CAD build for the part. Positions are in the model's coordinates, mm. A direction names the side the tool comes from. Give positions to 0.01 mm unless a question says otherwise; leave off trailing zeros. Loops run counter-clockwise (first coordinate to the right, second up) from the corner with the lowest first, then second, coordinate; pieces in that order, holes last. Notation, with made-up numbers: M 38.25,7 L 64.25,7 A27 cw 64.25,25 Z; hole C 44.5,53 d4. An arc over 180 degrees is marked long. Answer as CSV lines item,"result".
from build123d import *

# Parameters (mm, degrees)
SKETCH_W        = 43.2
SKETCH_H        = 46
SKETCH_W_2      = 31.5
SKETCH_H_2      = 34
PAD_DEPTH       = 41
SKETCH001_W     = 43.2
SKETCH001_H     = 46
SKETCH001_W_2   = 39.6
SKETCH001_H_2   = 42.4
PAD001_DEPTH    = 30
POCKET_DEPTH    = 5
SKETCH003_W     = 14
SKETCH003_H     = 12
PAD002_DEPTH    = 14
FILLET_R        = 6.99
POCKET001_DEPTH = 10
POCKET002_DEPTH = 43.201
SKETCH006_R     = 2
POCKET003_DEPTH = 2.001
SKETCH007_W     = 14
SKETCH007_H     = 12
PAD003_DEPTH    = 14
FILLET001_R     = 6.99
POCKET004_DEPTH = 10
POCKET005_DEPTH = 43.201
SKETCH010_R     = 2
POCKET006_DEPTH = 2.001


with BuildPart() as part:
    # Sketch → Pad (new body)
    with BuildSketch(Plane.XY):
        Rectangle(SKETCH_W, SKETCH_H)
        Rectangle(SKETCH_W_2, SKETCH_H_2, mode=Mode.SUBTRACT)
    extrude(amount=PAD_DEPTH)

    # Sketch001 → Pad001 (new body)
    with BuildSketch(Plane.XY.offset(41)):
        Rectangle(SKETCH001_W, SKETCH001_H)
        Rectangle(SKETCH001_W_2, SKETCH001_H_2, mode=Mode.SUBTRACT)
    extrude(amount=PAD001_DEPTH)

    # Sketch002 → Pocket (cut)
    with BuildSketch(Plane(origin=(-21.6, 0, 0), x_dir=(0, -1, 0), z_dir=(-1, 0, 0))):
        with BuildLine():
            Line((-11.5, 71), (11.5, 71))
            Line((11.5, 71), (11.5, 62.000009))
            ThreePointArc((-11.5, 61.999999), (5e-06, 50.5), (11.5, 62.000009))
            Line((-11.5, 61.999999), (-11.5, 71))
        make_face()
    extrude(amount=-POCKET_DEPTH, mode=Mode.SUBTRACT)

    # Sketch003 → Pad002 (new body)
    with BuildSketch(Plane.XZ.offset(23)):
        with Locations((-14.6, 6)):
            Rectangle(SKETCH003_W, SKETCH003_H)
        with Locations((14.6, 6)):
            Rectangle(SKETCH003_W, SKETCH003_H)
    extrude(amount=PAD002_DEPTH)

    # Fillet
    fillet_edges = [part.edges().sort_by_distance(p)[0] for p in [
        (-21.6, -37, 6),
        (-7.6, -37, 6),
        (7.6, -37, 6),
        (21.6, -37, 6),
    ]]
    fillet(fillet_edges, radius=FILLET_R)

    # Sketch004 → Pocket001 (cut)
    with BuildSketch(Plane.XY.offset(12)):
        with BuildLine():
            Line((-19.6, -23), (-9.6, -23))
            Line((-9.6, -23), (-9.6, -30.009996))
            ThreePointArc((-19.6, -30.009995), (-14.6, -35.009995), (-9.6, -30.009996))
            Line((-19.6, -30.009995), (-19.6, -23))
        make_face()
        with BuildLine():
            Line((9.6, -23), (19.6, -23))
            Line((19.6, -23), (19.6, -30.009994))
            ThreePointArc((9.6, -30.009994), (14.6, -35.009995), (19.6, -30.009994))
            Line((9.6, -30.009994), (9.6, -23))
        make_face()
    extrude(amount=-POCKET001_DEPTH, mode=Mode.SUBTRACT)

    # Sketch005 → Pocket002 (cut, through all)
    with BuildSketch(Plane(origin=(-21.6, 0, 0), x_dir=(0, -1, 0), z_dir=(-1, 0, 0))):
        Polygon((23, 12), (37, 2), (37, 12), align=None)
    extrude(amount=-POCKET002_DEPTH, mode=Mode.SUBTRACT)

    # Sketch006 → Pocket003 (cut, through all)
    with BuildSketch(Plane.XY.offset(2)):
        with Locations((-14.6, -30.009995)):
            Circle(SKETCH006_R)
        with Locations((14.6, -30.009995)):
            Circle(SKETCH006_R)
    extrude(amount=-POCKET003_DEPTH, mode=Mode.SUBTRACT)

    # Sketch007 → Pad003 (new body)
    with BuildSketch(Plane(origin=(0, 23, 0), x_dir=(-1, 0, 0), z_dir=(0, 1, 0))):
        with Locations((-14.6, 6)):
            Rectangle(SKETCH007_W, SKETCH007_H)
        with Locations((14.6, 6)):
            Rectangle(SKETCH007_W, SKETCH007_H)
    extrude(amount=PAD003_DEPTH)

    # Fillet001
    fillet001_edges = [part.edges().sort_by_distance(p)[0] for p in [
        (21.6, 37, 6),
        (7.6, 37, 6),
        (-7.6, 37, 6),
        (-21.6, 37, 6),
    ]]
    fillet(fillet001_edges, radius=FILLET001_R)

    # Sketch008 → Pocket004 (cut)
    with BuildSketch(Plane.XY.offset(12)):
        with BuildLine():
            Line((-19.6, 23), (-9.6, 23))
            Line((-9.6, 23), (-9.6, 30.009983))
            ThreePointArc((-9.6, 30.009983), (-14.6, 35.009995), (-19.6, 30.009983))
            Line((-19.6, 30.009983), (-19.6, 23))
        make_face()
        with BuildLine():
            Line((19.6, 30.009983), (19.6, 23))
            Line((19.6, 23), (9.6, 23))
            Line((9.6, 23), (9.6, 30.009983))
            ThreePointArc((19.6, 30.009983), (14.6, 35.009995), (9.6, 30.009983))
        make_face()
    extrude(amount=-POCKET004_DEPTH, mode=Mode.SUBTRACT)

    # Sketch009 → Pocket005 (cut, through all)
    with BuildSketch(Plane(origin=(-21.6, 0, 0), x_dir=(0, -1, 0), z_dir=(-1, 0, 0))):
        Polygon((-23, 12), (-37, 2), (-37, 12), align=None)
    extrude(amount=-POCKET005_DEPTH, mode=Mode.SUBTRACT)

    # Sketch010 → Pocket006 (cut, through all)
    with BuildSketch(Plane.XY.offset(2)):
        with Locations((-14.6, 30.009995)):
            Circle(SKETCH010_R)
        with Locations((14.6, 30.009995)):
            Circle(SKETCH010_R)
    extrude(amount=-POCKET006_DEPTH, mode=Mode.SUBTRACT)


solid = part.part
1) Band-saw the part on A-A on y = 0. Give the cut face in (x, z), and give its area (3 significant figures).
Answer below:
outline,"M -21.6,0 L -15.75,0 L -15.75,41 L -19.8,41 L -19.8,50.5 L -21.6,50.5 Z; M 15.75,0 L 21.6,0 L 21.6,71 L 19.8,71 L 19.8,41 L 15.75,41 Z"
area,"551 mm^2"
2) Flat gauge pins, fed straight in: pin 1 (2 mm diameter, centred on x = 4, z = 54, fed in from -Y); pin 2 (4.5 mm diameter, centred on x = -14.6, y = 30.01, fed in from +Z); pin 3 (3 mm diameter, centred on x = 14.6, y = 30.01, fed in from +Z); pin 4 (6 mm diameter, centred on x = -1.5, y = -17.5, fed in from +Z). Where does each tip first touch, or does it go through?
Answer below:
pin 1,"stops at y = -23"
pin 2,"stops at z = 2"
pin 3,"passes through"
pin 4,"stops at z = 41"
3) Mould opens along X. For faces 4 (the face through (7.6, 26, 5)), 5 (the face through (-13.525, 31.696, 1.014)), 6 (the face through (19.753, 31.004, 6.283)), 7 (the face through (20.38, 33.956, 1.991)) say: +X half, -X half, draft (parallel to the pull), parting line (faces both ways), or undercut.
Answer below:
face 4,"undercut"
face 5,"undercut"
face 6,"draft"
face 7,"+X half"
4) Band-saw the part on C-C on z = 14. Give the cut face in (x, y), and give its area (3 significant figures).
Answer below:
outline,"M -21.6,-23 L 21.6,-23 L 21.6,23 L -21.6,23 Z; hole M -15.75,-17 L 15.75,-17 L 15.75,17 L -15.75,17 Z"
area,"916 mm^2"
5) Band-saw the part on D-D on y = -19.5. Give the cut face in (x, z), and give its area (3 significant figures).
Answer below:
outline,"M -21.6,0 L 21.6,0 L 21.6,71 L 19.8,71 L 19.8,41 L -19.8,41 L -19.8,71 L -21.6,71 Z"
area,"1,880 mm^2"
6) Band-saw the part on B-B on x = 0.5. Give the cut face in (y, z), and give its area (3 significant figures).
Answer below:
outline,"M -23,0 L -17,0 L -17,41 L -21.2,41 L -21.2,71 L -23,71 Z; M 17,0 L 23,0 L 23,71 L 21.2,71 L 21.2,41 L 17,41 Z"
area,"600 mm^2"
7) Which spindle directions (+Z, -Z, +X, -X, +Y, -Y) get a long thin tool onto all of the face, cutting with end or side? Do faces 1 (the face through (-14.49, 35.01, 2.87)), 2 (the face through (-8.909, 34.082, 1.991)), 3 (the face through (15.75, 0, 20)). Say none if no direction does.
Answer below:
face 1,"+Z"
face 2,"+Z, -Z, +Y"
face 3,"+Z, -Z"
8) Drill centre lines: line 1 (Y direction, x = -14.6, z = 1.3); line 2 (X direction, y = -9, z = 49); line 3 (Y direction, x = 4.5, z = 20.5). Where is each one in solid material? Low to high. Write a range as from..to.
Answer below:
line 1,"y = -37..-32.01, -28.01..-17, 17..28.01, 32.01..37"
line 2,"x = -21.6..-19.8, 19.8..21.6"
line 3,"y = -23..-17, 17..23"
